Can you work these out from the model? Positions are in its coordinate system, mm. A direction names the side the tool comes from. Give positions to 0.01 mm unless a question says otherwise; leave off trailing zeros. Loops run counter-clockwise (first coordinate to the right, second up) from the corner with the lowest first, then second, coordinate; pieces in that order, holes last. Notation, with made-up numbers: (24, 18.25) -> (70, 18.25) arc R27 ccw to (70, 40.25) -> close; hole circle Ø11 at (-31.75, 19). An arc over 180 degrees is marked (long way). Use CSV: the item, a comma, the result in double quotes.
from build123d import *

# Parameters (mm, degrees)
HOLE_WIZARD_1_D = 9
CHAMFER_1_SIZE  = 1


with BuildPart() as part:
    # 草图1 → 旋转1 (revolve)
    with BuildSketch(Plane(origin=(0, 0, 0), x_dir=(0, 0, -1), z_dir=(1, 0, 0)), mode=Mode.PRIVATE) as revolve_1_sk:
        Polygon((0, 0), (0, 118), (37, 118), (37, 95), (45, 95), (45, 99), (48, 99), (48, 0), align=None)
    revolve(revolve_1_sk.sketch.rotate(Axis((0, 0, -48), (0, 0, 1)), 90), axis=Axis((0, 0, -48), (0, 0, 1)))

    # 草图2 → 切除-旋转1 (revolve, cut)
    with BuildSketch(Plane(origin=(0, 0, 0), x_dir=(0, 0, -1), z_dir=(1, 0, 0)), mode=Mode.PRIVATE) as cut_revolve_1_sk:
        Polygon((48, 0), (48, 91), (11, 91), (11, 56), (12.5, 56), (12.5, 45), (38.75, 45), (38.75, 0), align=None)
    revolve(cut_revolve_1_sk.sketch.rotate(Axis((0, 0, 0), (0, 0, -1)), 90), axis=Axis((0, 0, 0), (0, 0, -1)), mode=Mode.SUBTRACT)

    # 草图3 → 切除-旋转2 (revolve, cut)
    with BuildSketch(Plane(origin=(0, 0, 0), x_dir=(0, 0, -1), z_dir=(1, 0, 0)), mode=Mode.PRIVATE) as cut_revolve_2_sk:
        Polygon((0, 0), (0, 17), (3.5, 17), (3.5, 19.5), (7.5, 19.5), (7.5, 30), (19.75, 30), (19.75, 36), (38.75, 36), (38.75, 0), align=None)
    revolve(cut_revolve_2_sk.sketch.rotate(Axis((0, 0, 0), (0, 0, -1)), 90), axis=Axis((0, 0, 0), (0, 0, -1)), mode=Mode.SUBTRACT)

    # 孔1 (through all)
    with Locations(Plane(origin=(0, 0, -37), x_dir=(-1, 0, 0), z_dir=(0, 0, -1))):
        with Locations((54, 93.530743609), (108, 0), (54, -93.530743609), (-54, -93.530743609), (-108, 0), (-54, 93.530743609)):
            Hole(HOLE_WIZARD_1_D / 2)

    # 倒角1
    chamfer_1_edges = [part.edges().sort_by_distance(p)[0] for p in [
        (-30, 0, -19.75),
        (-36, 0, -38.75),
    ]]
    chamfer(chamfer_1_edges, length=CHAMFER_1_SIZE)


solid = part.part
(1) Which directions (+Z, -Z, +X, -X, +Y, -Y) give clear straight access to the entire face, cutting with the end or side of a thin tool? Please do faces 1 (the face through (-88, -37, -45)), 2 (the face through (103.504, 0.198, -18.241)), 3 (the face through (86.8, -27.33, -29.24)).
Answer sheet:
face 1,"none"
face 2,"+Z, -Z"
face 3,"-Z"
(2) If we section it at B-B, the plane z = -33.5: Give the number of separate pieces and of enclosed holes in the cut face, then the cut area to 3 significant figures.
Answer sheet:
separate pieces,"2"
enclosed holes,"8"
area,"19,600 mm2"
(3) If I drill on L1, parallel to X at y = 17.5, z = -30.5; L2, parallel to Y at x = 0, z = -1.9; L3, parallel to X at y = -95, z = -26.5, over which ranges is the centre line in solid material (lowest first)? Write a range as from..to.
Answer sheet:
L1,"x = -116.7..-89.3, -41.46..-31.46, 31.46..41.46, 89.3..116.7"
L2,"y = -118..-17, 17..118"
L3,"x = -69.99..-58.25, -49.75..49.75, 58.25..69.99"
(4) If we section it at A-A, the plane x = 108: Write out the boundary of the cut face in (y, z), then the cut area to 3 significant figures.
Answer sheet:
outline,"(-47.54, -37) -> (-4.5, -37) -> (-4.5, 0) -> (-47.54, 0) -> close; (4.5, -37) -> (47.54, -37) -> (47.54, 0) -> (4.5, 0) -> close"
area,"3,180 mm2"
(5) Will these pins go through, and if not, where does the flat tip stop? pin 1 Ø4 at (y, z) = (37.5, -8) entering from +X; pin 2 Ø3 at (x, y) = (-72, -89) entering from -Z; pin 3 Ø8 at (x, y) = (-108, 0) entering from +Z; pin 4 Ø19.5 at (x, y) = (-5, -6) entering from -Z.
Answer sheet:
pin 1,"stops at x = 112.53"
pin 2,"stops at z = -37"
pin 3,"passes through"
pin 4,"stops at z = -3.5"
(6) If we section it at D-D, the plane x = 79.5: Write out the boundary of the cut face in (y, z).
Answer sheet:
outline,"(-87.2, -37) -> (-52.01, -37) -> (-52.01, -45) -> (-59, -45) -> (-59, -48) -> (-44.28, -48) -> (-44.28, -11) -> (44.28, -11) -> (44.28, -48) -> (59, -48) -> (59, -45) -> (52.01, -45) -> (52.01, -37) -> (87.2, -37) -> (87.2, 0) -> (-87.2, 0) -> close"
(7) We'd pull the mould along X, two halves only. Please class faces 4 (the face through (20.59, 92.74, -41.06)), 5 (the face through (0, -46, -12.5)), 6 (the face through (25, -2, 0)): released by +X, released by -X, zero draft, split by the parting line, or undercut.
Answer sheet:
face 4,"split by the parting line"
face 5,"undercut"
face 6,"zero draft"
(8) If we section it at C-C, the plane y = -85.5: Write out the boundary of the cut face in (x, z), then the cut area to 3 significant figures.
Answer sheet:
outline,"(-81.32, -37) -> (-41.41, -37) -> (-41.41, -45) -> (-49.91, -45) -> (-49.91, -48) -> (-31.16, -48) -> (-31.16, -11) -> (31.16, -11) -> (31.16, -48) -> (49.91, -48) -> (49.91, -45) -> (41.41, -45) -> (41.41, -37) -> (81.32, -37) -> (81.32, 0) -> (-81.32, 0) -> close"
area,"4,670 mm2"
